from build123d import *

# Parameters (mm, degrees)
SKETCH_2_R      = 4
EXTRUDE_1_DEPTH = 35
CHAMFER_1_SIZE  = 1


with BuildPart() as part:
    # Эскиз2 → Бобышка-Вытянуть1 (new body)
    with BuildSketch(Plane(origin=(0, 0, 0), x_dir=(0, 0, -1), z_dir=(1, 0, 0))):
        Polygon((-10.969655115, 0), (-5.484827557, 9.5), (5.484827557, 9.5), (10.969655115, 0), (5.484827557, -9.5), (-5.484827557, -9.5), align=None)
        Circle(SKETCH_2_R, mode=Mode.SUBTRACT)
    extrude(amount=EXTRUDE_1_DEPTH)

    # Фаска1
    chamfer_1_edges = [part.edges().sort_by_distance(p)[0] for p in [
        (0, 0, 4),
        (35, 0, 4),
    ]]
    chamfer(chamfer_1_edges, length=CHAMFER_1_SIZE)


solid = part.part
Build history of the part. All positions in model axes, mm. Round coordinates to 2 decimals unless told otherwise and drop trailing zeros. Write each loop counter-clockwise with the first axis right and the second up, starting at its lowest first coordinate (ties: lowest second). Pieces come first, ordered by that corner, then holes. Notation, with made-up numbers: (-8, 70) - (5, 70) arc R33 cw to (5, 100) - close; hole circle Ø2 at (75, 1). An arc over 180 degrees is marked (long way). One line per question, with ' | ' between items.
1. Band-saw the part on B-B, the plane z = 0. Write the cut outline in (x, y).
Results are:
outline: (0, -9.5) - (35, -9.5) - (35, -5) - (34, -4) - (1, -4) - (0, -5) - close; (0, 5) - (1, 4) - (34, 4) - (35, 5) - (35, 9.5) - (0, 9.5) - close
2. Drop flat-ended pins along their axis: pin 1 Ø5 at (x, y) = (19.5, 4) entering from +Z; pin 2 Ø1.5 at (x, z) = (28, 8) entering from +Y; pin 3 Ø8 at (x, y) = (25.5, 5) entering from -Z. Give the stop position or say it passes through.
Results are:
pin 1: z = 10.1 | pin 2: y = 6.44 | pin 3: z = -10.39
3. Drill centre lines: line 1 along Y through (x, z) = (16.5, 0); line 2 along Z through (x, y) = (29.5, -1.5); line 3 along Y through (x, z) = (26, 3.5). Where is each one in solid material? Low to high. Write a range as from..to.
Results are:
line 1: -9.5..-4, 4..9.5 | line 2: -10.1..-3.71, 3.71..10.1 | line 3: -9.5..-1.94, 1.94..9.5
4. Mould opens along Y. For faces 1 (the face through (17, -9.5, 0)), 2 (the face through (35, 2, 5)), 3 (the face through (17.269, -3.905, 0.867)) say: released by +Y, released by -Y, zero draft, split by the parting line, or undercut.
Results are:
face 1: released by -Y | face 2: zero draft | face 3: undercut
5. Band-saw the part on D-D, the plane z = -7.75. Write the cut outline in (x, y), and give its area (3 significant figures).
Results are:
outline: (0, -5.58) - (35, -5.58) - (35, 5.58) - (0, 5.58) - close | area: 390 mm^2
6. Band-saw the part on C-C, the plane y = -7.25. Write the cut outline in (x, z), and give its area (3 significant figures).
Results are:
outline: (0, -6.78) - (35, -6.78) - (35, 6.78) - (0, 6.78) - close | area: 475 mm^2
7. Band-saw the part on A-A, the plane x = 21. Write the cut outline in (y, z).
Results are:
outline: (-9.5, -5.48) - (0, -10.97) - (9.5, -5.48) - (9.5, 5.48) - (0, 10.97) - (-9.5, 5.48) - close; hole circle Ø8 at (0, 0)
